Read the model definition and answer for the solid it produces. Units are mm, in the model's axes. A direction names the side the tool comes from. Coordinates: 2 decimals unless noted, no trailing zeros. Loops run counter-clockwise (first coordinate to the right, second up) from the corner with the lowest first, then second, coordinate; pieces in that order, holes last. Notation, with made-up numbers: M -16.75,-0.5 L -8.75,-0.5 A10 ccw -8.75,9.5 Z; hole C -26.75,89.5 d6. An arc over 180 degrees is marked long. Use one line per item in the form item = value. Start each with the question number.
1. For a pull along Z with two mould halves and no side action, classify faces 4 (the cylindrical face through (28.638, -90.264, -9.949)), 5 (the flat face through (26.34, -41, 4)), 6 (the cylindrical face through (28.638, -90.165, -0.969)) as released by +Z, released by -Z, zero draft, split by the parting line, or undercut.
2. Find the intervals of material crossed by probe 1 along X at (y, z) = (-56.5, 49); probe 2 along Z at (x, y) = (5, -16); probe 3 along Y at (x, z) = (-29.5, -47) (3 decimals), in increasing order. Write a range as [from, to].
3. The part is cut by section D-D (y = -84). Give the vertices of the cut face in (x, z).
4. The part is cut by section A-A (x = 12). Give the vertices of the cut face in (y, z) (3 decimals).
5. The part is cut by section B-B (y = -9). Give the vertices of the cut face in (x, z).
6. The part is cut by section C-C (z = -48). Give the vertices of the cut face in (x, y) (3 decimals), plus the area to 3 significant figures.
7. Flat-ended cylindrical pins translate along their axes: pin 1 (1 mm diameter, centred on x = -12, z = 7, fed in from -Y) (3 decimals); pin 2 (14 mm diameter, centred on y = -87.5, z = -5, fed in from -X); pin 3 (2 mm diameter, centred on x = 28.5, y = -83, fed in from -Z); pin 4 (1 mm diameter, centred on x = -18.5, z = 46, fed in from +Y). Find the tip coordinate at first contact, or state that the pin passes through.
8. A tool of negligible diameter and unlimited length cuts with its end or side. For faces 1 (the flat face through (27.737, -81, -7)), 2 (the flat face through (-46.685, -41, 2)), 3 (the flat face through (29.515, -45, 2)), from which of +Z, -Z, +X, -X, +Y, -Y can it reach the whole face along a straight path? Write none if from no direction.
from build123d import *

# Parameters (mm, degrees)
F0_W     = 79.375
F0_H     = 127
F1_DEPTH = 3.175
F2_W     = 73.025
F2_H     = 3.175
F3_DEPTH = 76.2
F4_W     = 1.778
F4_H     = 12.7
F5_DEPTH = 12.7
F6_R     = 6.35
F7_R     = 6.34999
F8_R     = 4.445
F9_DEPTH = 25.4


# Not quite as in the source:
# - a fillet or chamfer is up to 0.001 mm smaller than in the source, because OpenCascade refuses the exact size


with BuildPart() as f1:
    # F0 (on Front) → F1 (new body)
    with BuildSketch(Plane.XZ):
        with Locations((-10.1727880716, 3.2072235078)):
            Rectangle(F0_W, F0_H)
    extrude(amount=F1_DEPTH)

    # F2 (on face) → F3 (join)
    with BuildSketch(Plane.XZ.offset(3.175)):
        Polygon((-46.6852880716, 63.5322235078), (-46.6852880716, 66.7072235078), (-49.8602880716, 66.7072235078), (-49.8602880716, -60.2927764922), (-46.6852880716, -60.2927764922), (-46.6852880716, -57.1177764922), align=None)
        with Locations((-10.1727880716, 65.1197235078)):
            Rectangle(F2_W, F2_H)
        Polygon((29.5147119284, 66.7072235078), (26.3397119284, 66.7072235078), (26.3397119284, 63.5322235078), (26.3397119284, -57.1177764922), (26.3397119284, -60.2927764922), (29.5147119284, -60.2927764922), align=None)
        with Locations((-10.1727880716, -58.7052764922)):
            Rectangle(F2_W, F2_H)
    extrude(amount=F3_DEPTH)

    # F4 (on face) → F5 (join)
    with BuildSketch(Plane.XZ.offset(79.375)):
        with Locations((28.6257119284, -5.5081006922)):
            Rectangle(F4_W, F4_H)
    extrude(amount=F5_DEPTH)

    # F6
    f6_edges = [f1.edges().sort_by_distance(p)[0] for p in [
        (28.625712, -92.075, 0.841899),
    ]]
    fillet(f6_edges, radius=F6_R)

    # F7 (radius 6.35 in the source; OpenCascade refuses exactly that, so slightly less here)
    f7_edges = [f1.edges().sort_by_distance(p)[0] for p in [
        (28.625712, -92.075, -11.858101),
    ]]
    fillet(f7_edges, radius=F7_R)

    # F8 (on face) → F9 (cut)
    with BuildSketch(Plane.YZ.offset(29.5147119284)):
        with Locations((-85.725, -5.5081006922)):
            Circle(F8_R)
    extrude(amount=-F9_DEPTH, mode=Mode.SUBTRACT)


solid = f1.part
Computed values:
q1.face_4 = released by -Z
q1.face_5 = undercut
q1.face_6 = released by +Z
q2.probe_1 = [-49.86, -46.69], [26.34, 29.51]
q2.probe_2 = [-60.29, -57.12], [63.53, 66.71]
q2.probe_3 = [-3.175, 0]
q3.outline = M 27.74,-11.86 L 29.51,-11.86 L 29.51,-9.6 L 27.74,-9.6 Z; M 27.74,-1.41 L 29.51,-1.41 L 29.51,0.84 L 27.74,0.84 Z
q4.outline = M -79.375,-60.293 L 0,-60.293 L 0,66.707 L -79.375,66.707 L -79.375,63.532 L -3.175,63.532 L -3.175,-57.118 L -79.375,-57.118 Z
q5.outline = M -49.86,-60.29 L 29.51,-60.29 L 29.51,66.71 L -49.86,66.71 Z; hole M -46.69,-57.12 L 26.34,-57.12 L 26.34,63.53 L -46.69,63.53 Z
q6.outline = M -49.86,-79.375 L -46.685,-79.375 L -46.685,-3.175 L 26.34,-3.175 L 26.34,-79.375 L 29.515,-79.375 L 29.515,0 L -49.86,0 Z
q6.area = 736 mm²
q7.pin_1 = -3.175
q7.pin_2 = 27.74
q7.pin_3 = -11.86
q7.pin_4 = 0
q8.face_1 = +Z, -Z, -X, -Y
q8.face_2 = -Y
q8.face_3 = +Z, -Z, +X, +Y, -Y
